The model under review builds one solid part; all positions refer to its coordinate system, in mm. Round coordinates to 2 decimals unless told otherwise and drop trailing zeros. Loops run counter-clockwise (first coordinate to the right, second up) from the corner with the lowest first, then second, coordinate; pieces in that order, holes last. Notation, with made-up numbers: M -2,6 L 7,6 A15 cw 7,27 Z; hole C 85.5,17.5 d9. An arc over 180 degrees is marked long. Return JSON: item names as keys, results as strings. Group by question number.
Q1. Draft analysis for pull direction X (two halves, no side actions). For faces 1 (the face through (-109, 10, -21.793)), 2 (the face through (-206.424, 1.69, -13.123)), state which applies: pulls with the +X half, pulls with the -X half, needs draft (parallel to the pull), parting line crosses it, or undercut.
Q2. To check wall thickness, follow line 1 along X through (y, z) = (16.9, -12.7); line 2 along Y through (x, z) = (-144, -8); line 3 along Z through (x, y) = (-203.2, 18). State the ranges of each line that lie inside material, in increasing order.
Q3. Consider section C-C (x = -12.7). State the section outline as (y, z) points.
Q4. Clearance check with flat-ended pins moving along their axes: pin 1 Ø1.1 at (y, z) = (8, -24.5) entering from +X; pin 2 Ø6 at (x, z) = (-60, -6.5) entering from -Y; pin 3 Ø6.5 at (x, y) = (-120, 10.5) entering from +Z; pin 4 Ø3 at (y, z) = (10, -24) entering from -X. State where each tip first meets the part, or that it passes through.
Q5. Consider section B-B (z = -12.7). State the section outline as (x, y) points.
Q6. Consider section D-D (x = -141). State the section outline as (y, z) points.
Q7. Consider section A-A (x = 22.5). State the section outline as (y, z) points, and give its area (3 significant figures).
Autodesk Inventor part; units mm, degrees
ref_plane "YZ Plane" through (0, 0, 0) normal (1, 0, 0) x (0, 1, 0)
ref_plane "XZ Plane" through (0, 0, 0) normal (0, 1, 0) x (-1, 0, 0)
ref_plane "XY Plane" through (0, 0, 0) normal (0, 0, 1) x (1, 0, 0)
sketch "Sketch1" plane through (0, 0, 0) normal (0, 1, 0) x (-1, 0, 0)
  line L0 (0, 0) -> (431.8, 0)
  line L1 (431.8, 0) -> (431.8, -25.4)
  line L2 (431.8, -25.4) -> (0, -25.4)
  line L3 (0, -25.4) -> (0, 0)
  dimension "d0" = 431.8
  dimension "d1" = 25.4
extrude "Extrusion1" add sketch "Sketch1" along normal blind 3.429
sketch "Sketch2" plane through (0, 3.429, 0) normal (0, 1, 0) x (1, 0, 0)
  line L0 (0, 25.4) -> (-431.8, 25.4)
  line L1 (-44.45, 25.4) -> (-171.0436, 25.4)
  line L2 (-171.0436, 25.4) -> (-171.0436, 21.7932)
  line L3 (-171.0436, 21.7932) -> (-44.45, 21.7932)
  line L4 (-44.45, 21.7932) -> (-44.45, 25.4)
  line L5 (0, 0) -> (0, 25.4)
  point P0 (-44.45, 23.5966)
  dimension "d4" = 126.5936
  dimension "d5" = 3.6068
  dimension "d6" = 44.45
extrude "Extrusion2" add sketch "Sketch2" along normal blind 12.5984
sketch "Sketch3" plane through (0, 16.0274, 0) normal (0, 1, 0) x (1, 0, 0)
  line L0 (-431.8, 0) -> (0, 0)
  line L1 (0, 0) -> (0, 25.4)
  line L2 (0, 25.4) -> (-431.8, 25.4)
  line L3 (-431.8, 25.4) -> (-431.8, 0)
extrude "Extrusion3" add sketch "Sketch3" along normal blind 3.429
sketch "Sketch4" plane through (0, 19.4564, 0) normal (0, 1, 0) x (1, 0, 0)
  line L0 (0, 25.4) -> (-431.8, 25.4)
  line L1 (0, 0) -> (0, 25.4)
  line L2 (-431.8, 25.4) -> (-431.8, 0)
  point P0 (-12.7, 12.7)
  point P1 (-419.1, 12.7)
  point P2 (-203.2, 12.7)
  dimension "d11" = 12.7
  dimension "d12" = 12.7
  dimension "d13" = 12.7
  dimension "d14" = 12.7
  dimension "d15" = 12.7
  dimension "d16" = 203.2
hole "Hole1" at (-12.7, 19.4564, -12.7) at (-203.2, 19.4564, -12.7) direction (0, -1, 0) diameter 6.5024 end through all
sketch "Sketch6" plane through (0, 0, 0) normal (0, -1, 0) x (1, 0, 0)
  circle A0 centre (-203.2, -12.7) radius 3.2512
  circle A1 centre (-12.7, -12.7) radius 3.2512
  line L0 (0, -25.4) -> (-431.8, -25.4)
  line L1 (0, 0) -> (0, -25.4)
  line L2 (-431.8, 0) -> (0, 0)
  line L3 (-431.8, -25.4) -> (-431.8, 0)
  line L4 (-431.8, -25.4) -> (-254, -25.4)
  line L5 (-254, -25.4) -> (-254, 0)
  line L6 (-254, 0) -> (-431.8, 0)
  line L7 (-431.8, 0) -> (-431.8, -25.4)
  dimension "d26" = 177.8
extrude "Extrusion5" cut sketch "Sketch6" against normal blind 76.2 contours L0 L3 L2 L5
sketch "Sketch7" plane through (0, 0, 0) normal (1, 0, 0) x (0, 0, -1)
  line L0 (0, 0) -> (25.4, 0)
  line L1 (25.4, 0) -> (25.4, 3.429)
  line L2 (0, 3.429) -> (25.4, 3.429)
  line L3 (0, 0) -> (0, 3.429)
  line L4 (0, 16.0274) -> (25.4, 16.0274)
  line L5 (25.4, 16.0274) -> (25.4, 19.4564)
  line L6 (0, 19.4564) -> (25.4, 19.4564)
  line L7 (0, 16.0274) -> (0, 19.4564)
extrude "Extrusion6" add sketch "Sketch7" along normal blind 76.2
properties part number "ArmPart2"
Values:
{
 "1": {"face 1": "needs draft", "face 2": "undercut"},
 "2": {"line 1": "x = -254 to -206.45, -199.95 to -15.95, -9.45 to 76.2", "line 2": "y = 0 to 3.43, 16.03 to 19.46", "line 3": "z = -25.4 to -15.95, -9.45 to 0"},
 "3": {"outline": "M 0,-25.4 L 3.43,-25.4 L 3.43,-15.95 L 0,-15.95 Z; M 0,-9.45 L 3.43,-9.45 L 3.43,0 L 0,0 Z; M 16.03,-25.4 L 19.46,-25.4 L 19.46,-15.95 L 16.03,-15.95 Z; M 16.03,-9.45 L 19.46,-9.45 L 19.46,0 L 16.03,0 Z"},
 "4": {"pin 1": "stops at x = -44.45", "pin 2": "stops at y = 0", "pin 3": "stops at z = -21.79", "pin 4": "stops at x = -171.04"},
 "5": {"outline": "M -254,0 L -206.45,0 L -206.45,3.43 L -254,3.43 Z; M -254,16.03 L -206.45,16.03 L -206.45,19.46 L -254,19.46 Z; M -199.95,0 L -15.95,0 L -15.95,3.43 L -199.95,3.43 Z; M -199.95,16.03 L -15.95,16.03 L -15.95,19.46 L -199.95,19.46 Z; M -9.45,0 L 76.2,0 L 76.2,3.43 L -9.45,3.43 Z; M -9.45,16.03 L 76.2,16.03 L 76.2,19.46 L -9.45,19.46 Z"},
 "6": {"outline": "M 0,-25.4 L 19.46,-25.4 L 19.46,0 L 16.03,0 L 16.03,-21.79 L 3.43,-21.79 L 3.43,0 L 0,0 Z"},
 "7": {"outline": "M 0,-25.4 L 3.43,-25.4 L 3.43,0 L 0,0 Z; M 16.03,-25.4 L 19.46,-25.4 L 19.46,0 L 16.03,0 Z", "area": "174 mm2"}
}
